Read the model definition and answer for the solid it produces. Units are mm, in the model's axes. A direction names the side the tool comes from. Coordinates: 2 decimals unless noted, no trailing zeros. Loops run counter-clockwise (first coordinate to the right, second up) from the corner with the lowest first, then second, coordinate; pieces in that order, holes last. Notation, with made-up numbers: (74.25, 7) -> (129.25, 7) arc R20 cw to (129.25, 37) -> close; hole circle Ø1 at (41.5, 6.25). An arc over 180 degrees is marked (long way). Answer in a Markdown table with one row per item.
```python
from build123d import *

# Parameters (mm, degrees)
SKETCH1_R           = 1.5
BOSS_EXTRUDE1_DEPTH = 1.7
BOSS_EXTRUDE2_DEPTH = 3
BOSS_EXTRUDE3_DEPTH = 0.5
CUT_EXTRUDE2_REACH  = 39.314
SKETCH4_R           = 0.230396576


with BuildPart() as part:
    # Sketch1 → Boss-Extrude1 (new body)
    with BuildSketch(Plane(origin=(0, 0, 0), x_dir=(1, 0, 0), z_dir=(0, 1, 0))):
        with BuildLine():
            Line((-16, 18), (16, 18))
            ThreePointArc((16, 18), (17.414213562, 17.414213562), (18, 16))
            Line((18, 16), (18, -16))
            ThreePointArc((18, -16), (17.414213562, -17.414213562), (16, -18))
            Line((16, -18), (-16, -18))
            ThreePointArc((-16, -18), (-17.414213562, -17.414213562), (-18, -16))
            Line((-18, -16), (-18, 16))
            ThreePointArc((-18, 16), (-17.414213562, 17.414213562), (-16, 18))
        make_face()
        with Locations(Location((-15.25, 15.25, 0), (0, 0, 270))):
            Circle(SKETCH1_R, mode=Mode.SUBTRACT)
        with Locations(Location((15.25, 15.25, 0), (0, 0, 270))):
            Circle(SKETCH1_R, mode=Mode.SUBTRACT)
        with Locations(Location((-15.25, -15.25, 0), (0, 0, 270))):
            Circle(SKETCH1_R, mode=Mode.SUBTRACT)
        with Locations(Location((15.25, -15.25, 0), (0, 0, 270))):
            Circle(SKETCH1_R, mode=Mode.SUBTRACT)
    extrude(amount=BOSS_EXTRUDE1_DEPTH)

    # Sketch2 → Boss-Extrude2 (add)
    with BuildSketch(Plane.XY.offset(18)):
        with BuildLine():
            Line((8.220977072, 1.7), (12.220977072, 1.7))
            Line((12.220977072, 1.7), (12.220977072, 2.791290101))
            ThreePointArc((12.220977072, 2.791290101), (12.162398428, 2.932711457), (12.020977072, 2.991290101))
            Line((12.020977072, 2.991290101), (11.710977072, 2.991290101))
            ThreePointArc((11.710977072, 2.991290101), (11.569555715, 3.049868744), (11.510977072, 3.191290101))
            Line((11.510977072, 3.191290101), (11.510977072, 3.271290101))
            ThreePointArc((11.510977072, 3.271290101), (11.452398428, 3.412711457), (11.310977072, 3.471290101))
            Line((11.310977072, 3.471290101), (9.010977072, 3.471290101))
            ThreePointArc((9.010977072, 3.471290101), (8.869555715, 3.412711457), (8.810977072, 3.271290101))
            Line((8.810977072, 3.271290101), (8.810977072, 3.191290101))
            ThreePointArc((8.810977072, 3.191290101), (8.752398428, 3.049868744), (8.610977072, 2.991290101))
            Line((8.610977072, 2.991290101), (8.420977072, 2.991290101))
            ThreePointArc((8.420977072, 2.991290101), (8.279555715, 2.932711457), (8.220977072, 2.791290101))
            Line((8.220977072, 2.791290101), (8.220977072, 1.7))
        make_face()
        with BuildLine():
            Line((8.320977072, 1.8), (12.120977072, 1.8))
            Line((12.120977072, 1.8), (12.120977072, 2.791290101))
            ThreePointArc((12.120977072, 2.791290101), (12.09168775, 2.862000779), (12.020977072, 2.891290101))
            Line((12.020977072, 2.891290101), (11.710977072, 2.891290101))
            ThreePointArc((11.710977072, 2.891290101), (11.498845037, 2.979158066), (11.410977072, 3.191290101))
            Line((11.410977072, 3.191290101), (11.410977072, 3.271290101))
            ThreePointArc((11.410977072, 3.271290101), (11.38168775, 3.342000779), (11.310977072, 3.371290101))
            Line((11.310977072, 3.371290101), (9.010977072, 3.371290101))
            ThreePointArc((9.010977072, 3.371290101), (8.940266393, 3.342000779), (8.910977072, 3.271290101))
            Line((8.910977072, 3.271290101), (8.910977072, 3.191290101))
            ThreePointArc((8.910977072, 3.191290101), (8.823109106, 2.979158066), (8.610977072, 2.891290101))
            Line((8.610977072, 2.891290101), (8.420977072, 2.891290101))
            ThreePointArc((8.420977072, 2.891290101), (8.350266393, 2.862000779), (8.320977072, 2.791290101))
            Line((8.320977072, 2.791290101), (8.320977072, 1.8))
        make_face(mode=Mode.SUBTRACT)
    extrude(amount=-BOSS_EXTRUDE2_DEPTH)

    # Sketch3 → Boss-Extrude3 (add)
    with BuildSketch(Plane(origin=(0, 0, 15), x_dir=(-1, 0, 0), z_dir=(0, 0, -1))):
        with BuildLine():
            Line((-8.220977072, 1.7), (-8.220977072, 2.791290101))
            ThreePointArc((-8.220977072, 2.791290101), (-8.279555715, 2.932711457), (-8.420977072, 2.991290101))
            Line((-8.420977072, 2.991290101), (-8.610977072, 2.991290101))
            ThreePointArc((-8.610977072, 2.991290101), (-8.752398428, 3.049868744), (-8.810977072, 3.191290101))
            Line((-8.810977072, 3.191290101), (-8.810977072, 3.271290101))
            ThreePointArc((-8.810977072, 3.271290101), (-8.869555715, 3.412711457), (-9.010977072, 3.471290101))
            Line((-9.010977072, 3.471290101), (-11.310977072, 3.471290101))
            ThreePointArc((-11.310977072, 3.471290101), (-11.452398428, 3.412711457), (-11.510977072, 3.271290101))
            Line((-11.510977072, 3.271290101), (-11.510977072, 3.191290101))
            ThreePointArc((-11.510977072, 3.191290101), (-11.569555715, 3.049868744), (-11.710977072, 2.991290101))
            Line((-11.710977072, 2.991290101), (-12.020977072, 2.991290101))
            ThreePointArc((-12.020977072, 2.991290101), (-12.162398428, 2.932711457), (-12.220977072, 2.791290101))
            Line((-12.220977072, 2.791290101), (-12.220977072, 1.7))
            Line((-12.220977072, 1.7), (-8.220977072, 1.7))
        make_face()
    extrude(amount=BOSS_EXTRUDE3_DEPTH)

    # Sketch4 → Cut-Extrude2 (cut, up to next)
    with BuildSketch(Plane(origin=(0, 0, 14.5), x_dir=(-1, 0, 0), z_dir=(0, 0, -1)), mode=Mode.PRIVATE) as cut_extrude2_sk1:
        with Locations((-11.120977072, 2.671290101)):
            Circle(SKETCH4_R)
    cut_extrude2_tool1 = extrude(cut_extrude2_sk1.sketch, amount=-CUT_EXTRUDE2_REACH, mode=Mode.PRIVATE) & part.part
    # Sketch4 → Cut-Extrude2 (cut, up to next)
    with BuildSketch(Plane(origin=(0, 0, 14.5), x_dir=(-1, 0, 0), z_dir=(0, 0, -1)), mode=Mode.PRIVATE) as cut_extrude2_sk2:
        with Locations((-10.420977072, 2.671290101)):
            Circle(SKETCH4_R)
    cut_extrude2_tool2 = extrude(cut_extrude2_sk2.sketch, amount=-CUT_EXTRUDE2_REACH, mode=Mode.PRIVATE) & part.part
    # Sketch4 → Cut-Extrude2 (cut, up to next)
    with BuildSketch(Plane(origin=(0, 0, 14.5), x_dir=(-1, 0, 0), z_dir=(0, 0, -1)), mode=Mode.PRIVATE) as cut_extrude2_sk3:
        with Locations((-9.720977072, 2.671290101)):
            Circle(SKETCH4_R)
    cut_extrude2_tool3 = extrude(cut_extrude2_sk3.sketch, amount=-CUT_EXTRUDE2_REACH, mode=Mode.PRIVATE) & part.part
    add(cut_extrude2_tool1.solids().sort_by_distance((11.120977, 2.67129, 14.5))[0], mode=Mode.SUBTRACT)
    add(cut_extrude2_tool2.solids().sort_by_distance((10.420977, 2.67129, 14.5))[0], mode=Mode.SUBTRACT)
    add(cut_extrude2_tool3.solids().sort_by_distance((9.720977, 2.67129, 14.5))[0], mode=Mode.SUBTRACT)


solid = part.part
```
1. Given pin 1 Ø4 at (x, z) = (-15.25, -15.25) entering from +Y; pin 2 Ø5 at (x, z) = (15.25, 15.25) entering from -Y; pin 3 Ø0.5 at (y, z) = (2, 16) entering from -X, each flat-ended and moving along its own axis, determine where each tip first touches the part or whether it passes through.
A:
| item | result |
|---|---|
| pin 1 | stops at y = 1.7 |
| pin 2 | stops at y = 0 |
| pin 3 | stops at x = 8.22 |
2. A cutting plane is placed at C-C on y = 1.25. Give the vertices of the cut face in (x, z), and give its area (3 significant figures).
A:
| item | result |
|---|---|
| outline | (-18, -16) arc R2 ccw to (-16, -18) -> (16, -18) arc R2 ccw to (18, -16) -> (18, 16) arc R2 ccw to (16, 18) -> (-16, 18) arc R2 ccw to (-18, 16) -> close; hole circle Ø3 at (-15.25, -15.25); hole circle Ø3 at (-15.25, 15.25); hole circle Ø3 at (15.25, -15.25); hole circle Ø3 at (15.25, 15.25) |
| area | 1,260 mm2 |
3. A cutting plane is placed at B-B on x = 15.25. Give the vertices of the cut face in (y, z), and give its area (3 significant figures).
A:
| item | result |
|---|---|
| outline | (0, -18) -> (1.7, -18) -> (1.7, -16.75) -> (0, -16.75) -> close; (0, -13.75) -> (1.7, -13.75) -> (1.7, 13.75) -> (0, 13.75) -> close; (0, 16.75) -> (1.7, 16.75) -> (1.7, 18) -> (0, 18) -> close |
| area | 51.0 mm2 |
4. A tool of negligible diameter and unlimited length cuts with its end or side. For faces 5 (the cylindrical face through (-15.18, 0.84, -16.75)), 6 (the flat face through (10, 1.8, 17)), from which of +Z, -Z, +X, -X, +Y, -Y can it reach the whole face along a straight path? Write none if from no direction.
A:
| item | result |
|---|---|
| face 5 | +Y, -Y |
| face 6 | +Z |
5. The mould has two halves that part along Z. Classify faces 1 (the flat face through (0, 0, 0)), 2 (the flat face through (0, 1, 18)), 3 (the flat face through (0, 1, -18)), 4 (the cylindrical face through (-15.18, 0.84, 13.75)): pulls with the +Z half, pulls with the -Z half, needs draft (parallel to the pull), parting line crosses it, or undercut.
A:
| item | result |
|---|---|
| face 1 | needs draft |
| face 2 | pulls with the +Z half |
| face 3 | pulls with the -Z half |
| face 4 | undercut |
6. Find the intervals of material crossed by probe 1 along X at (y, z) = (0.4, 15.25); probe 2 along Y at (x, z) = (-14.5, -8); probe 3 along Z at (x, y) = (14.5, 1.45), in increasing order.
A:
| item | result |
|---|---|
| probe 1 | x = -18 to -16.75, -13.75 to 13.75, 16.75 to 18 |
| probe 2 | y = 0 to 1.7 |
| probe 3 | z = -18 to -16.55, -13.95 to 13.95, 16.55 to 18 |
7. A cutting plane is placed at D-D on z = -3. Give the vertices of the cut face in (x, y).
A:
| item | result |
|---|---|
| outline | (-18, 0) -> (18, 0) -> (18, 1.7) -> (-18, 1.7) -> close |
8. A cutting plane is placed at A-A on z = -15.25. Give the vertices of the cut face in (x, y), and give its area (3 significant figures).
A:
| item | result |
|---|---|
| outline | (-18, 0) -> (-16.75, 0) -> (-16.75, 1.7) -> (-18, 1.7) -> close; (-13.75, 0) -> (13.75, 0) -> (13.75, 1.7) -> (-13.75, 1.7) -> close; (16.75, 0) -> (18, 0) -> (18, 1.7) -> (16.75, 1.7) -> close |
| area | 51.0 mm2 |
